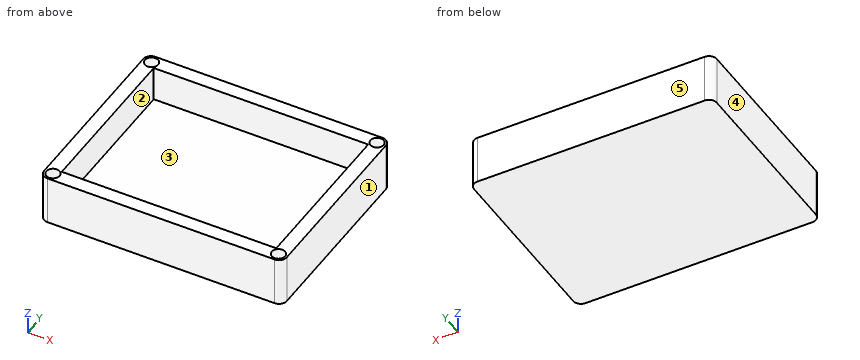
Autodesk Fusion 360 part; units mm, degrees
sketch "Sketch1" plane through (0, 0, 0) normal (0, 0, 1) x (1, 0, 0) in component "part 1"
  line L0 (-15.5, 12.25) -> (15.5, 12.25)
  line L1 (15.5, 12.25) -> (15.5, -12.25)
  line L2 (15.5, -12.25) -> (-15.5, -12.25)
  line L3 (-15.5, -12.25) -> (-15.5, 12.25)
  line L4 (-15.5, 12.25) -> (15.5, -12.25) construction
  line L5 (15.5, 12.25) -> (-15.5, -12.25) construction
  dimension "d1" = 31
  dimension "d2" = 24.5
extrude "Extrude1" add sketch "Sketch1" along normal blind 6.3 in component "part 1"
sketch "Sketch2" plane through (0, 0, 6.3) normal (0, 0, 1) x (-1, 0, 0) in component "part 1"
  line L0 (15.5, 12.25) -> (-15.5, 12.25)
  line L1 (-15.5, 12.25) -> (-15.5, -12.25)
  line L2 (-15.5, -12.25) -> (15.5, -12.25)
  line L3 (15.5, -12.25) -> (15.5, 12.25)
shell "Shell1" thickness 1.8 removed faces 1 at (-5.1667, 4.0833, 6.3) in component "part 1"
sketch "Sketch3" plane through (0, 0, 6.3) normal (0, 0, 1) x (-1, 0, 0) in component "part 1"
  circle A0 centre (14.4, -11.2) radius 0.85
  line L0 (0, 0) -> (0, -3.5)
  line L1 (0, 0) -> (3.5, 0)
  circle A1 centre (-14.4, -11.2) radius 0.85
  circle A2 centre (-14.4, 11.2) radius 0.85
  circle A3 centre (14.4, 11.2) radius 0.85
  dimension "d8" = 1.7
  dimension "d9" = 11.2
  dimension "d10" = 14.4
extrude "Extrude2" cut sketch "Sketch3" against normal blind 4 in component "part 1"
fillet "Fillet1" radius 1 1 edges at (15.5, -12.25, 3.15) in component "part 1"
fillet "Fillet1" radius 1 1 edges at (15.5, 12.25, 3.15) in component "part 1"
fillet "Fillet1" radius 1 1 edges at (-15.5, 12.25, 3.15) in component "part 1"
fillet "Fillet1" radius 1 1 edges at (-15.5, -12.25, 3.15) in component "part 1"
component "part 1" placed x (1, 0, 0) y (0, 1, 0) z (0, 0, 1) at (0, 0, 0)
Could you check a few things on this model? Use its own coordinates, in mm. Face numbers are marked on the shaded views. A direction names the side the tool comes from. Coordinates: 2 decimals unless noted, no trailing zeros. Loops run counter-clockwise (first coordinate to the right, second up) from the corner with the lowest first, then second, coordinate; pieces in that order, holes last. Notation, with made-up numbers: (-18.75, 45.25) -> (7.25, 45.25) arc R26 ccw to (7.25, 77.25) -> close; hole circle Ø5 at (-23, -36.5). An arc over 180 degrees is marked (long way). Answer in a Markdown table with one row per item.
(1) Imagine slicing it at C-C (x = -7.5). List the corners of the cut face in (y, z) for me.
Results found:
| item | result |
|---|---|
| outline | (-12.25, 0) -> (12.25, 0) -> (12.25, 6.3) -> (10.45, 6.3) -> (10.45, 1.8) -> (-10.45, 1.8) -> (-10.45, 6.3) -> (-12.25, 6.3) -> close |
(2) Imagine slicing it at A-A (z = 5.25). List the corners of the cut face in (x, y) for me.
Results found:
| item | result |
|---|---|
| outline | (-15.5, -11.25) arc R1 ccw to (-14.5, -12.25) -> (14.5, -12.25) arc R1 ccw to (15.5, -11.25) -> (15.5, 11.25) arc R1 ccw to (14.5, 12.25) -> (-14.5, 12.25) arc R1 ccw to (-15.5, 11.25) -> close; hole circle Ø1.7 at (-14.4, -11.2); hole circle Ø1.7 at (-14.4, 11.2); hole (-13.7, -10.45) -> (13.7, -10.45) -> (13.7, 10.45) -> (-13.7, 10.45) -> close; hole circle Ø1.7 at (14.4, -11.2); hole circle Ø1.7 at (14.4, 11.2) |
(3) Thinking about a two-plate mould opening in Y: for the marked faces 3, 4 and 5, which applies, released by +Y, released by -Y, zero draft, split by the parting line, or undercut?
Results found:
| item | result |
|---|---|
| face 3 | undercut |
| face 4 | zero draft |
| face 5 | released by +Y |
(4) Will these pins go through, and if not, where does the flat tip stop? pin 1 Ø1.4 at (x, y) = (-14.5, 11) entering from +Z; pin 2 Ø8 at (x, y) = (3.5, 3.5) entering from +Z.
Results found:
| item | result |
|---|---|
| pin 1 | stops at z = 6.3 |
| pin 2 | stops at z = 1.8 |
(5) For the marked faces 1 and 2, which set-ups out of +Z, -Z, +X, -X, +Y, -Y let a thin tool reach every point of the face, with its end or its side?
Results found:
| item | result |
|---|---|
| face 1 | +Z, -Z, +X, +Y, -Y |
| face 2 | +Z |
(6) Imagine slicing it at B-B (y = 1.25). List the corners of the cut face in (x, z) for me, plus the area to 3 significant figures.
Results found:
| item | result |
|---|---|
| outline | (-15.5, 0) -> (15.5, 0) -> (15.5, 6.3) -> (13.7, 6.3) -> (13.7, 1.8) -> (-13.7, 1.8) -> (-13.7, 6.3) -> (-15.5, 6.3) -> close |
| area | 72.0 mm^2 |
(7) If I drill on probe 1 along X at (y, z) = (11.2, 5.3); probe 2 along Y at (x, z) = (14.4, 4.9); probe 3 along Y at (x, z) = (-7.5, 4), over which ranges is the centre line in solid material (lowest first)?
Results found:
| item | result |
|---|---|
| probe 1 | x = -15.5 to -15.25, -13.55 to 13.55, 15.25 to 15.5 |
| probe 2 | y = -12.25 to -12.05, -10.35 to 10.35, 12.05 to 12.25 |
| probe 3 | y = -12.25 to -10.45, 10.45 to 12.25 |
